Design review of the part shown in the three views and the two pictorial views. Dimensions are in mm from the part's minimum x, y and z. Coordinates: 2 decimals unless noted, no trailing zeros. One line per item, written item: value. Start each with the question number.
(1) To check wall thickness, follow line 1 along Z through (x, y) = (448.5, 5); line 2 along Z through (x, y) = (467, 6); line 3 along X through (y, z) = (4, 68). State the ranges of each line that lie inside material, in increasing order.
(2) Consider section A-A on y = 3.75. Count the separate pieces of the cut face and the enclosed holes in it, then the cut area to 3 significant figures.
(3) Clearance check with flat-ended pins moving along their axes: pin 1 (5 mm diameter, centred on y = 5, z = 352.5, fed in from -X); pin 2 (6 mm diameter, centred on x = 540, z = 352, fed in from -Y); pin 3 (2.5 mm diameter, centred on x = 472, z = 30, fed in from +Y); pin 4 (5 mm diameter, centred on y = 3.5, z = 352.5, fed in from +X). State where each tip first meets the part, or that it passes through.
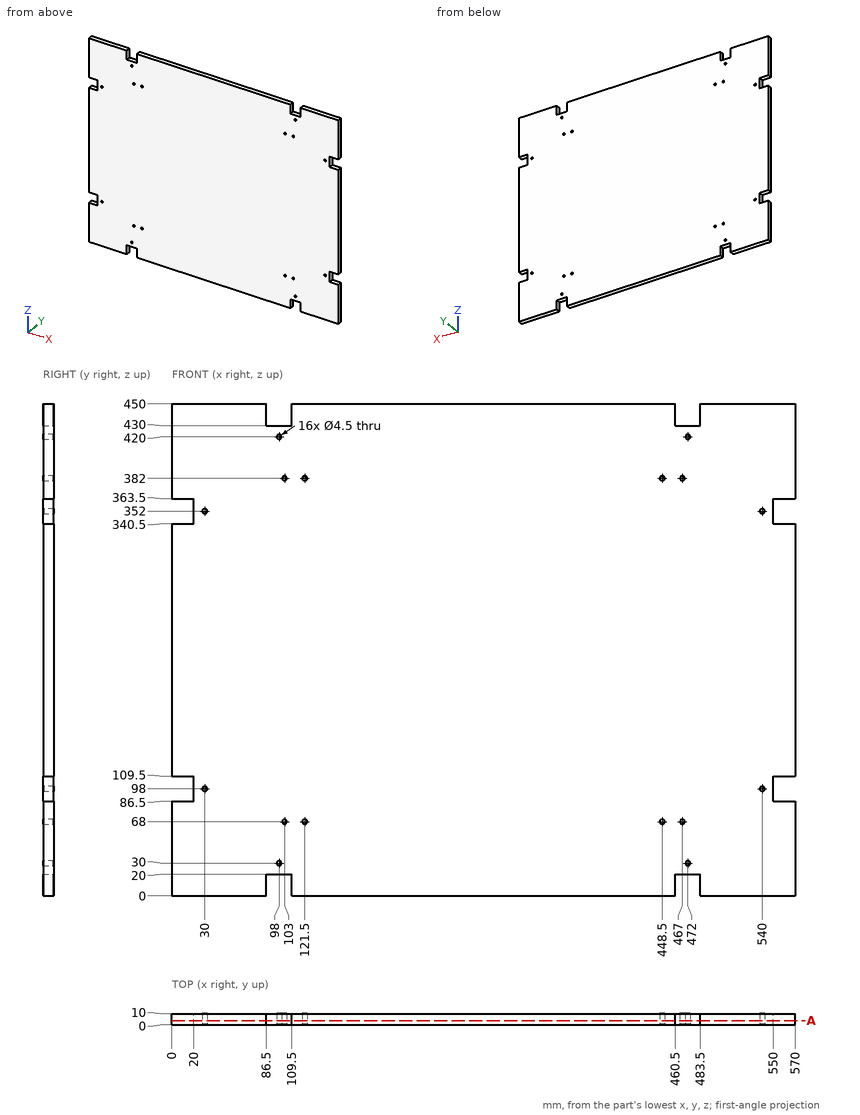
Geometry check:
1. line 1: z = 0 to 65.75, 70.25 to 379.75, 384.25 to 450
1. line 2: z = 20 to 65.75, 70.25 to 379.75, 384.25 to 430
1. line 3: x = 0 to 100.75, 105.25 to 119.25, 123.75 to 446.25, 450.75 to 464.75, 469.25 to 570
2. separate pieces: 1
2. enclosed holes: 16
2. area: 253,000 mm^2
3. pin 1: stops at x = 20
3. pin 2: stops at y = 0
3. pin 3: passes through
3. pin 4: stops at x = 550
